Could you check a few things on this model? Use its own coordinates, in mm. Face numbers are marked on the shaded views. A direction names the side the tool comes from. Give positions to 0.01 mm unless a question says otherwise; leave off trailing zeros. Order: outer loops, then holes, each group sorted by start corner. A loop starts at its lowest first (then second) coordinate and runs counter-clockwise, first axis right, second up.
(1) Imagine slicing it at B-B, the plane z = 6.5. Write out the boundary of the cut face in (x, y).
(2) If we mould it in two halves opening along Y, with no side actions, what happens to the marked faces 1, 2 and 3? For each: released by +Y, released by -Y, zero draft, split by the parting line, or undercut.
(3) On a 3-axis mill with a long thin cutter (end or side, diameter ignored), from which of +Z, -Z, +X, -X, +Y, -Y can I reach the whole of each face in a straight line? I mean the marked faces 4, 5 and 6. Say none if no direction works.
(4) Will these pins go through, and if not, where does the flat tip stop? pin 1 (5 mm diameter, centred on x = 0, y = -2, fed in from +Z); pin 2 (3 mm diameter, centred on y = 3, z = 7.5, fed in from +X); pin 3 (2 mm diameter, centred on x = 4.5, z = 3.5, fed in from -Y); pin 4 (4 mm diameter, centred on x = 0, z = 6.5, fed in from +Y).
(5) Imagine slicing it at C-C, the plane y = 2. Write out the boundary of the cut face in (x, z).
(6) If I drill on probe 1 along Z at (x, y) = (4.7, 0); probe 2 along Z at (x, y) = (-7.5, -2.25); probe 3 along Y at (x, z) = (0.25, 3.75), over which ranges is the centre line in solid material (lowest first)?
(7) Imagine slicing it at A-A, the plane x = 0. Write out the boundary of the cut face in (y, z), then the cut area to 3 significant figures.
(8) Imagine slicing it at D-D, the plane x = 1.75. Write out the boundary of the cut face in (y, z), then the cut area to 3 significant figures.
from build123d import *

# Parameters (mm, degrees)
SKETCH_1_R                       = 8.5
EXTRUDE_1_DEPTH                  = 3
SKETCH_2_R                       = 6
EXTRUDE_2_DEPTH                  = 7
CUT_EXTRUDE_1_REACH              = 17.636
SKETCH_3_R                       = 4
HOLE_WIZARD_M3_1_REACH           = 20.021
HOLE_WIZARD_M3_1_BORE_R          = 1.25
HOLE_WIZARD_M3_1_ON_FACE_2_REACH = 20.021
HOLE_WIZARD_M3_1_BORE_2_R        = 1.25


with BuildPart() as part:
    # 스케치1 → 보스-돌출1 (new body)
    with BuildSketch(Plane.XY):
        Circle(SKETCH_1_R)
    extrude(amount=EXTRUDE_1_DEPTH)

    # 스케치2 → 보스-돌출2 (add)
    with BuildSketch(Plane.XY.offset(3)):
        Circle(SKETCH_2_R)
    extrude(amount=EXTRUDE_2_DEPTH)

    # 스케치3 → 컷-돌출1 (cut, up to next)
    with BuildSketch(Plane(origin=(0, 0, 0), x_dir=(-1, 0, 0), z_dir=(0, 0, -1)), mode=Mode.PRIVATE) as cut_extrude_1_sk1:
        Circle(SKETCH_3_R)
    cut_extrude_1_tool1 = extrude(cut_extrude_1_sk1.sketch, amount=-CUT_EXTRUDE_1_REACH, mode=Mode.PRIVATE) & part.part
    add(cut_extrude_1_tool1.solids().sort_by_distance((0, 0, 0))[0], mode=Mode.SUBTRACT)

    # M3 나사 구멍1 bore (on position points) → M3 나사 구멍1 (cut, up to next)
    with BuildSketch(Plane(origin=(0, 6, 6.5), x_dir=(1, 0, 0), z_dir=(0, 1, 0)), mode=Mode.PRIVATE) as hole_wizard_m3_1_sk1:
        Circle(HOLE_WIZARD_M3_1_BORE_R)
    hole_wizard_m3_1_tool1 = extrude(hole_wizard_m3_1_sk1.sketch, amount=-HOLE_WIZARD_M3_1_REACH, mode=Mode.PRIVATE) & part.part
    add(hole_wizard_m3_1_tool1.solids().sort_by_distance((0, 6, 6.5))[0], mode=Mode.SUBTRACT)

    # M3 나사 구멍1 bore 2 (on position points) → M3 나사 구멍1 on face 2 (cut, up to next)
    with BuildSketch(Plane(origin=(6, 0, 6.5), x_dir=(0, 0, 1), z_dir=(1, 0, 0)), mode=Mode.PRIVATE) as hole_wizard_m3_1_on_face_2_sk1:
        Circle(HOLE_WIZARD_M3_1_BORE_2_R)
    hole_wizard_m3_1_on_face_2_tool1 = extrude(hole_wizard_m3_1_on_face_2_sk1.sketch, amount=-HOLE_WIZARD_M3_1_ON_FACE_2_REACH, mode=Mode.PRIVATE) & part.part
    add(hole_wizard_m3_1_on_face_2_tool1.solids().sort_by_distance((6, 0, 6.5))[0], mode=Mode.SUBTRACT)


solid = part.part
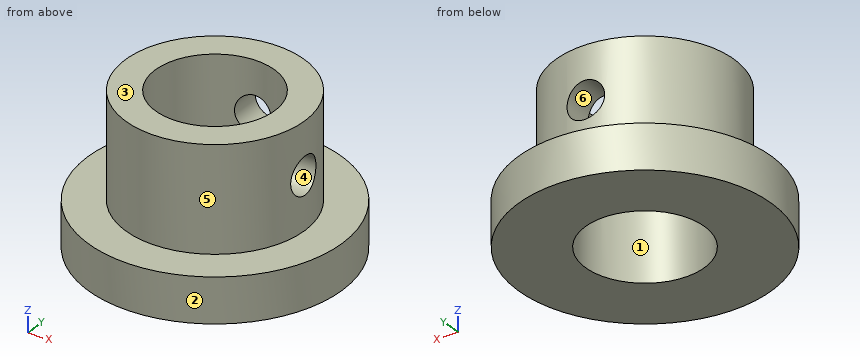
Answer block:
1. outline: (-1.25, 3.8) - (-1.25, 5.87) arc R6 ccw (long way) to (5.87, -1.25) - (3.8, -1.25) arc R4 cw (long way) to start; (1.25, 3.8) arc R4 cw to (3.8, 1.25) - (5.87, 1.25) arc R6 ccw to (1.25, 5.87) - close
2. face 1: undercut
2. face 2: split by the parting line
2. face 3: zero draft
3. face 4: +X
3. face 5: +Z
3. face 6: +Y
4. pin 1: stops at z = 10
4. pin 2: stops at x = 5.81
4. pin 3: stops at y = -7.68
4. pin 4: stops at y = 6
5. outline: (-8.26, 0) - (-3.46, 0) - (-3.46, 10) - (-5.66, 10) - (-5.66, 3) - (-8.26, 3) - close; (3.46, 0) - (8.26, 0) - (8.26, 3) - (5.66, 3) - (5.66, 10) - (3.46, 10) - close
6. probe 1: z = 0 to 5.25, 7.75 to 10
6. probe 2: z = 0 to 3
6. probe 3: y = -5.99 to -3.99, 3.99 to 5.99
7. outline: (-8.5, 0) - (-4, 0) - (-4, 10) - (-6, 10) - (-6, 3) - (-8.5, 3) - close; (4, 0) - (8.5, 0) - (8.5, 3) - (6, 3) - (6, 5.25) - (4, 5.25) - close; (4, 7.75) - (6, 7.75) - (6, 10) - (4, 10) - close
7. area: 50.0 mm2
8. outline: (-8.32, 0) - (-3.6, 0) - (-3.6, 10) - (-5.74, 10) - (-5.74, 3) - (-8.32, 3) - close; (3.6, 0) - (8.32, 0) - (8.32, 3) - (5.74, 3) - (5.74, 10) - (3.6, 10) - close
8. area: 58.3 mm2
